```python
from build123d import *

# Parameters (mm, degrees)
BOSS_EXTRUDE1_DEPTH          = 6.35
SKETCH2_W                    = 6.35
SKETCH2_H                    = 12.5
CUT_EXTRUDE1_DEPTH           = 117.791791236
F_10_0_1935_DIAMETER_HOLE2_D = 4.9149
SKETCH7_R                    = 3.24358
CUT_EXTRUDE2_DEPTH           = 117.791791236
FILLET1_R                    = 3


with BuildPart() as part:
    # Sketch1 → Boss-Extrude1 (new body)
    with BuildSketch(Plane(origin=(0, 0, 0), x_dir=(1, 0, 0), z_dir=(0, 1, 0))):
        Polygon((0, 0), (20, 0), (20, 57.3), (60, 57.3), (60, 82.7), (20, 82.7), (20, 100), (0, 100), align=None)
    extrude(amount=BOSS_EXTRUDE1_DEPTH)

    # Sketch2 → Cut-Extrude1 (cut, through all)
    with BuildSketch(Plane(origin=(0, 6.35, 0), x_dir=(1, 0, 0), z_dir=(0, 1, 0))):
        with Locations((10, 70)):
            Rectangle(SKETCH2_W, SKETCH2_H)
        with Locations((10, 30.5258)):
            Rectangle(SKETCH2_W, SKETCH2_H)
    extrude(amount=-CUT_EXTRUDE1_DEPTH, mode=Mode.SUBTRACT)

    # #10 (0.1935) Diameter Hole2 (through all)
    with Locations(Plane(origin=(0, 6.35, 0), x_dir=(1, 0, 0), z_dir=(0, 1, 0))):
        with Locations((10, 89.7371), (10, 50.2629), (10, 10.7887)):
            Hole(F_10_0_1935_DIAMETER_HOLE2_D / 2)

    # Sketch7 → Cut-Extrude2 (cut, through all)
    with BuildSketch(Plane(origin=(0, 6.35, 0), x_dir=(1, 0, 0), z_dir=(0, 1, 0))):
        with Locations(Location((25, 70, 0), (0, 0, 270))):
            Circle(SKETCH7_R)
        with Locations(Location((50.4, 70, 0), (0, 0, 270))):
            Circle(SKETCH7_R)
    extrude(amount=-CUT_EXTRUDE2_DEPTH, mode=Mode.SUBTRACT)

    # Fillet1
    fillet1_edges = [part.edges().sort_by_distance(p)[0] for p in [
        (0, 3.175, -100),
        (20, 3.175, -100),
        (60, 3.175, -82.7),
        (60, 3.175, -57.3),
        (20, 3.175, 0),
        (0, 3.175, 0),
    ]]
    fillet(fillet1_edges, radius=FILLET1_R)


solid = part.part
```
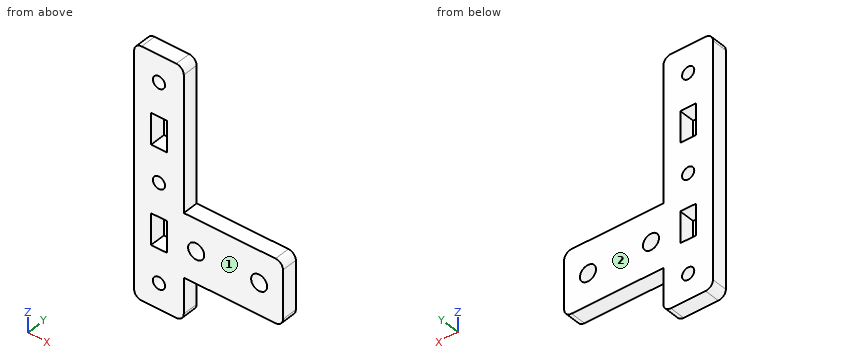
Source: CAD feature listing. Evaluate the final solid. Frame: model axes, mm. Face numbers are marked on the shaded views. Coordinates: 2 decimals unless noted, no trailing zeros. Loops run counter-clockwise (first coordinate to the right, second up) from the corner with the lowest first, then second, coordinate; pieces in that order, holes last. Notation, with made-up numbers: M 42.25,74 L 81.25,74 A21 ccw 81.25,80 Z; hole C 62.25,-12.75 d11. An arc over 180 degrees is marked long. Put each result on its own line as item: value. Start each with the question number.
1) Cut plane A-A on x = 25. Return the cut outline in (y, z).
2) Ray query, L1, parallel to Z at x = 10, y = 3.5; L2, parallel to X at y = 4.75, z = -70 (3 decimals); L3, parallel to X at y = 3.75, z = -89.5. Return the intervals inside material, ascending. Write a range as from..to.
3) Cut plane C-C on z = -70. Return the cut outline in (x, y) (3 decimals).
4) Cut plane D-D on y = 3. Return the cut outline in (x, z) (3 decimals), then the cut area to 3 significant figures.
5) Contact query for flat-ended pins moving along their axis: pin 1 Ø6 at (x, z) = (50.4, -70) entering from -Y; pin 2 Ø1.9 at (x, y) = (37.5, 2.5) entering from -Z; pin 3 Ø6.5 at (x, z) = (10, -50.26) entering from -Y; pin 4 Ø1.9 at (y, z) = (2.5, -93) entering from +X. Output: stop coordinate, or through.
6) Pull-direction query (Y, two-part tool) for the marked faces 1 and 2; classes: pulls with the +Y half, pulls with the -Y half, needs draft (parallel to the pull), parting line crosses it, or undercut.
7) Cut plane B-B on z = -29. Return the cut outline in (x, y) (3 decimals).
The answers:
1. outline: M 0,-82.7 L 6.35,-82.7 L 6.35,-73.24 L 0,-73.24 Z; M 0,-66.76 L 6.35,-66.76 L 6.35,-57.3 L 0,-57.3 Z
2. L1: z = -100..-92.19, -87.28..-76.25, -63.75..-52.72, -47.81..-36.78, -24.28..-13.25, -8.33..0
2. L2: x = 0..6.825, 13.175..21.756, 28.244..47.156, 53.644..60
2. L3: x = 0..7.55, 12.45..20
3. outline: M 0,0 L 6.825,0 L 6.825,6.35 L 0,6.35 Z; M 13.175,0 L 21.756,0 L 21.756,6.35 L 13.175,6.35 Z; M 28.244,0 L 47.156,0 L 47.156,6.35 L 28.244,6.35 Z; M 53.644,0 L 60,0 L 60,6.35 L 53.644,6.35 Z
4. outline: M 0,-97 A3 ccw 3,-100 L 17,-100 A3 ccw 20,-97 L 20,-82.7 L 57,-82.7 A3 ccw 60,-79.7 L 60,-60.3 A3 ccw 57,-57.3 L 20,-57.3 L 20,-3 A3 ccw 17,0 L 3,0 A3 ccw 0,-3 Z; hole M 6.825,-76.25 L 13.175,-76.25 L 13.175,-63.75 L 6.825,-63.75 Z; hole M 6.825,-36.776 L 13.175,-36.776 L 13.175,-24.276 L 6.825,-24.276 Z; hole C 10,-89.737 d4.915; hole C 10,-50.263 d4.915; hole C 10,-10.789 d4.915; hole C 25,-70 d6.487; hole C 50.4,-70 d6.487
4. area: 2,720 mm²
5. pin 1: passes through
5. pin 2: stops at z = -82.7
5. pin 3: stops at y = 0
5. pin 4: stops at x = 20
6. face 1: pulls with the -Y half
6. face 2: pulls with the +Y half
7. outline: M 0,0 L 6.825,0 L 6.825,6.35 L 0,6.35 Z; M 13.175,0 L 20,0 L 20,6.35 L 13.175,6.35 Z
